```python
from build123d import *

# Parameters (mm, degrees)
SKETCH1_R           = 1.5875
BOSS_EXTRUDE1_DEPTH = 1.5875
BOSS_EXTRUDE2_START = 1.5875
SKETCH1_3_W         = 5.9309
SKETCH1_3_H         = 12.7
SKETCH1_3_W_2       = 10.5691
BOSS_EXTRUDE2_DEPTH = 11
BOSS_EXTRUDE3_START = 1.5875
SKETCH1_4_W         = 10.286
SKETCH1_4_H         = 8.89
BOSS_EXTRUDE3_DEPTH = 6.5
BOSS_EXTRUDE4_START = 1.5875
SKETCH1_5_W         = 1.27
SKETCH1_5_H         = 8.89
SKETCH1_5_W_2       = 2.16
BOSS_EXTRUDE4_DEPTH = 10.86
SKETCH2_W           = 10.286
SKETCH2_H           = 4.445
REVOLVE1_ANGLE      = 180
SKETCH1_6_W         = 20.6629
SKETCH1_6_H         = 2.54
SKETCH1_6_W_2       = 5
SKETCH1_6_H_2       = 46.17
SKETCH1_6_W_3       = 25.4
BOSS_EXTRUDE5_DEPTH = 8.5


with BuildPart() as part:
    # Sketch1 → Boss-Extrude1 (new body)
    with BuildSketch(Plane(origin=(0, 0, 0), x_dir=(1, 0, 0), z_dir=(0, 1, 0))):
        Polygon((0, 0), (0, 53.34), (97, 53.34), (99, 51.34), (99, 41.95), (101.6, 39.35), (101.6, 4.35), (99, 1.75), (99, 0), align=None)
        with Locations((96.52, 2.54)):
            Circle(SKETCH1_R, mode=Mode.SUBTRACT)
        with Locations((71.074776633, 7.62)):
            Circle(SKETCH1_R, mode=Mode.SUBTRACT)
        with Locations((13.97, 2.54)):
            Circle(SKETCH1_R, mode=Mode.SUBTRACT)
        with Locations((15.24, 50.8)):
            Circle(SKETCH1_R, mode=Mode.SUBTRACT)
        with Locations((90.17, 50.8)):
            Circle(SKETCH1_R, mode=Mode.SUBTRACT)
    extrude(amount=BOSS_EXTRUDE1_DEPTH)

    # Sketch1<3> → Boss-Extrude2 (add)
    with BuildSketch(Plane(origin=(0, 0, 0), x_dir=(1, 0, 0), z_dir=(0, 1, 0)).offset(BOSS_EXTRUDE2_START)):
        with Locations((-2.96545, 37.99)):
            Rectangle(SKETCH1_3_W, SKETCH1_3_H)
        with Locations((5.28455, 37.99)):
            Rectangle(SKETCH1_3_W_2, SKETCH1_3_H)
    extrude(amount=BOSS_EXTRUDE2_DEPTH)

    # Sketch1<4> → Boss-Extrude3 (add)
    with BuildSketch(Plane(origin=(0, 0, 0), x_dir=(1, 0, 0), z_dir=(0, 1, 0)).offset(BOSS_EXTRUDE3_START)):
        with Locations((7.303, 8.763)):
            Rectangle(SKETCH1_4_W, SKETCH1_4_H)
    extrude(amount=BOSS_EXTRUDE3_DEPTH)

    # Sketch1<5> → Boss-Extrude4 (add)
    with BuildSketch(Plane(origin=(0, 0, 0), x_dir=(1, 0, 0), z_dir=(0, 1, 0)).offset(BOSS_EXTRUDE4_START)):
        with Locations((-0.635, 8.763)):
            Rectangle(SKETCH1_5_W, SKETCH1_5_H)
        with Locations((1.08, 8.763)):
            Rectangle(SKETCH1_5_W_2, SKETCH1_5_H)
    extrude(amount=BOSS_EXTRUDE4_DEPTH)

    # Sketch2 → Revolve1 (revolve)
    with BuildSketch(Plane(origin=(0, 8.0875, 0), x_dir=(1, 0, 0), z_dir=(0, 1, 0))):
        with Locations((7.303, 6.5405)):
            Rectangle(SKETCH2_W, SKETCH2_H)
    revolve(axis=Axis((2.16, 8.0875, -8.763), (-1, 0, 0)), revolution_arc=REVOLVE1_ANGLE)

    # Sketch1<6> → Boss-Extrude5 (add)
    with BuildSketch(Plane(origin=(0, 0, 0), x_dir=(1, 0, 0), z_dir=(0, 1, 0))):
        with Locations((58.90895, 2.54)):
            Rectangle(SKETCH1_6_W, SKETCH1_6_H)
        with Locations((81.95945, 2.54)):
            Rectangle(SKETCH1_6_W, SKETCH1_6_H)
        with Locations((94.7909, 28.985)):
            Rectangle(SKETCH1_6_W_2, SKETCH1_6_H_2)
        with Locations((35.85845, 2.54)):
            Rectangle(SKETCH1_6_W, SKETCH1_6_H)
        with Locations((76.87945, 50.8)):
            Rectangle(SKETCH1_6_W, SKETCH1_6_H)
        with Locations((53.82895, 50.8)):
            Rectangle(SKETCH1_6_W, SKETCH1_6_H)
        with Locations((30.0355, 50.8)):
            Rectangle(SKETCH1_6_W_3, SKETCH1_6_H)
    extrude(amount=BOSS_EXTRUDE5_DEPTH)


solid = part.part
```
Check sheet for the modelled part. Datum: model origin and axes. Units: mm. A direction names the side the tool comes from. Give positions to 0.01 mm unless a question says otherwise; leave off trailing zeros. Loops run counter-clockwise (first coordinate to the right, second up) from the corner with the lowest first, then second, coordinate; pieces in that order, holes last. Notation, with made-up numbers: M 59,74 L 116,74 A11 cw 116,88 Z; hole C -35.5,-30.75 d7. An arc over 180 degrees is marked long. Answer in a Markdown table with one row per item.
1) Cross-section at B-B (z = -30.5). Enter the section's corners in (x, y), plus the area to 3 significant figures.
Solutions:
| item | result |
|---|---|
| outline | M 0,0 L 101.6,0 L 101.6,1.59 L 97.29,1.59 L 97.29,8.5 L 92.29,8.5 L 92.29,1.59 L 0,1.59 Z |
| area | 196 mm^2 |
2) Cross-section at C-C (x = 5.5). Enter the section's corners in (y, z) (1 decimal), plus the area to 3 significant figures.
Solutions:
| item | result |
|---|---|
| outline | M 0,-53.3 L 1.6,-53.3 L 1.6,-44.3 L 12.6,-44.3 L 12.6,-31.6 L 1.6,-31.6 L 1.6,-13.2 L 8.1,-13.2 A4.4 ccw 8.1,-4.3 L 1.6,-4.3 L 1.6,0 L 0,0 Z |
| area | 313 mm^2 |
3) Tool access check on faces 4 (the face through (95, 5, -5.9)), 5 (the face through (59, 5, -1.27)), 6 (the face through (95, 8.5, -29)). Record the directions out of +Z, -Z, +X, -X, +Y, -Y that give a thin tool (end or side, any length) a straight path to the whole face; none if there is none.
Solutions:
| item | result |
|---|---|
| face 4 | +Z, +X, +Y |
| face 5 | +Z, +X, -X, +Y |
| face 6 | +Z, -Z, +X, +Y |
4) Thickness scan on line 1 (Z direction, x = 36.5, y = 6); line 2 (X direction, y = 1.2, z = -7.62); line 3 (X direction, y = 4, z = -3). Record the ranges inside material, lowest first.
Solutions:
| item | result |
|---|---|
| line 1 | z = -52.07 to -49.53, -3.81 to -1.27 |
| line 2 | x = 0 to 69.49, 72.66 to 101.6 |
| line 3 | x = 25.53 to 46.19, 48.58 to 69.24, 71.63 to 92.29 |
5) Cross-section at D-D (y = 3.5). Count the separate pieces of the cut face and the enclosed holes in it, plus the area to 3 significant figures.
Solutions:
| item | result |
|---|---|
| separate pieces | 9 |
| enclosed holes | 0 |
| area | 889 mm^2 |
6) Depth check by flat-ended pin: pin 1 (5.5 mm diameter, centred on x = 82.5, y = 6, fed in from -Z); pin 2 (4 mm diameter, centred on y = 9.5, z = -5.5, fed in from +X); pin 3 (0.8 mm diameter, centred on x = 33.5, z = -2.5, fed in from +Y). Enter the tip coordinate at first touch or a pass-through.
Solutions:
| item | result |
|---|---|
| pin 1 | stops at z = -52.07 |
| pin 2 | stops at x = 97.29 |
| pin 3 | stops at y = 8.5 |
7) Cross-section at A-A (x = 90.17). Enter the section's corners in (y, z).
Solutions:
| item | result |
|---|---|
| outline | M 0,-53.34 L 1.59,-53.34 L 1.59,-52.39 L 0,-52.39 Z; M 0,-49.21 L 1.59,-49.21 L 1.59,-3.81 L 8.5,-3.81 L 8.5,-1.27 L 1.59,-1.27 L 1.59,0 L 0,0 Z |
8) Mould release check, pull along X, two halves, no side actions. Record for faces 1 (the face through (30, 5, -52.07)), 2 (the face through (10.569, 7, -38)), 3 (the face through (100.28, 0.78, -40.67)): released by +X, released by -X, zero draft, split by the parting line, or undercut.
Solutions:
| item | result |
|---|---|
| face 1 | zero draft |
| face 2 | undercut |
| face 3 | released by +X |
